Source: CAD feature listing. Evaluate the final solid. Frame: model axes, mm. Face numbers are marked on the shaded views. Give positions to 0.01 mm unless a question says otherwise; leave off trailing zeros. Loops run counter-clockwise (first coordinate to the right, second up) from the corner with the lowest first, then second, coordinate; pieces in that order, holes last. Notation, with made-up numbers: M 34.25,-1 L 80.25,-1 A12 cw 80.25,12 Z; hole C 36.5,36 d5. An arc over 180 degrees is marked long. Answer in a Markdown table with one row per item.
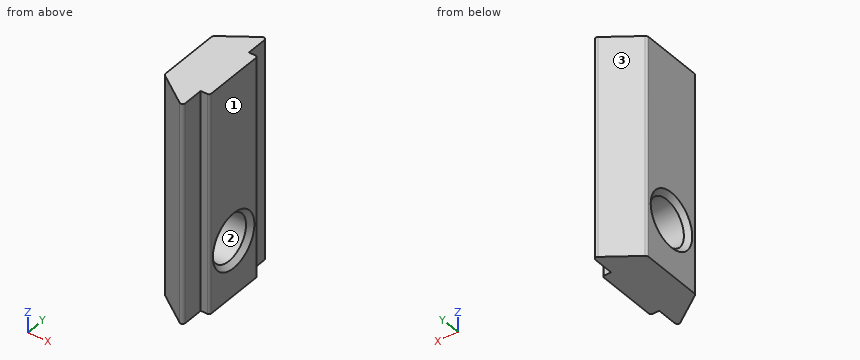
Autodesk Inventor part; units mm, degrees
ref_plane "nut_XY" through (0, 0, 0) normal (1, 0, 0) x (0, 0, -1)
ref_plane "nut_YZ" through (0, 0, 0) normal (0, 0, -1) x (0, 1, 0)
ref_plane "nut_ZX" through (0, 0, 0) normal (0, 1, 0) x (1, 0, 0)
sketch "Sketch_2" plane through (0, 0, 0) normal (0, 0, 1) x (1, 0, 0)
  arc A0 (-4.1, -2.7438) -> (-3.972, -2.9896) centre (-3.8, -2.7438) ccw
  line L0 (-3.972, -2.9896) -> (-1.1589, -4.9588)
  arc A1 (-1.1589, -4.9588) -> (-0.8, -4.7719) centre (-1.0281, -4.7719) ccw
  line L1 (-0.8, -4.7719) -> (-0.8, -2.9)
  line L2 (-0.8, -2.9) -> (-0.2, -2.9)
  arc A2 (-0.2, -2.9) -> (0, -2.7) centre (-0.2, -2.7) ccw
  line L3 (0, -2.7) -> (0, 2.7)
  arc A3 (0, 2.7) -> (-0.2, 2.9) centre (-0.2, 2.7) ccw
  line L4 (-0.2, 2.9) -> (-0.8, 2.9)
  line L5 (-0.8, 2.9) -> (-0.8, 4.7719)
  arc A4 (-0.8, 4.7719) -> (-1.1589, 4.9588) centre (-1.0281, 4.7719) ccw
  line L6 (-1.1589, 4.9588) -> (-3.972, 2.9896)
  arc A5 (-3.972, 2.9896) -> (-4.1, 2.7438) centre (-3.8, 2.7438) ccw
  line L7 (-4.1, 2.7438) -> (-4.1, -2.7438)
extrude "Extrusion1" add sketch "Sketch_2" along normal blind 15 and the other way blind 5
sketch "Sketch_5" plane through (0, 0, 0) normal (0, 0, 1) x (1, 0, 0)
  line L0 (0, 0) -> (-4.1, 0)
  line L1 (-4.1, 0) -> (-4.1, 2.5)
  line L2 (-4.1, 2.5) -> (-3.667, 2.067)
  line L3 (-3.667, 2.067) -> (-0.433, 2.067)
  line L4 (-0.433, 2.067) -> (0, 2.5)
  line L5 (0, 2.5) -> (0, 0)
  line L6 (0, 0) -> (-4.1, 0)
revolve "Revolution1" cut sketch "Sketch_5" angle 360 about axis through (0, 0, 0) along (1, 0, 0)
thread "Thread1"
ref_plane "nut_XY" through (0, 0, 0) normal (1, 0, 0) x (0, 0, -1)
ref_plane "nut_YZ" through (0, 0, 0) normal (0, 0, -1) x (0, 1, 0)
ref_plane "nut_ZX" through (0, 0, 0) normal (0, 1, 0) x (1, 0, 0)
ref_plane "to_bolt_XY" through (-4.1, 0, 0) normal (1, 0, 0) x (0, 0, -1)
ref_plane "to_bolt_YZ" through (-4.1, 0, 0) normal (0, 0, -1) x (0, 1, 0)
ref_plane "to_bolt_ZX" through (-4.1, 0, 0) normal (0, 1, 0) x (1, 0, 0)
ref_plane "to_frames_XY" through (-0.8, 0, 0) normal (1, 0, 0) x (0, 0, -1)
ref_plane "to_frames_YZ" through (-0.8, 0, 0) normal (0, 0, -1) x (0, 1, 0)
ref_plane "to_frames_ZX" through (-0.8, 0, 0) normal (0, 1, 0) x (1, 0, 0)
ref_plane "to_lane_XY" through (0, 0, 0) normal (0, 0, 1) x (1, 0, 0)
ref_plane "to_lane_YZ" through (0, 0, 0) normal (1, 0, 0) x (0, 1, 0)
ref_plane "to_lane_ZX" through (0, 0, 0) normal (0, 1, 0) x (0, 0, 1)
properties part number "HNTTSS5-5"
Q1. Section query B-B (z = 0). Output: boundary loops of the cut face in (x, y).
Values follow:
| item | result |
|---|---|
| outline | M -4.1,-2.74 A0.3 ccw -3.97,-2.99 L -1.16,-4.96 A0.23 ccw -0.8,-4.77 L -0.8,-2.9 L -0.2,-2.9 A0.2 ccw 0,-2.7 L 0,-2.5 L -0.43,-2.07 L -3.67,-2.07 L -4.1,-2.5 Z; M -4.1,2.5 L -3.67,2.07 L -0.43,2.07 L 0,2.5 L 0,2.7 A0.2 ccw -0.2,2.9 L -0.8,2.9 L -0.8,4.77 A0.23 ccw -1.16,4.96 L -3.97,2.99 A0.3 ccw -4.1,2.74 Z |
Q2. Section query D-D (x = -1.45). Output: boundary loops of the cut face in (y, z), plus the area to 3 significant figures.
Values follow:
| item | result |
|---|---|
| outline | M -4.76,-5 L 4.76,-5 L 4.76,15 L -4.76,15 Z; hole C 0,0 d4.13 |
| area | 177 mm^2 |
Q3. Contact query for flat-ended pins moving along their axis: pin 1 Ø2 at (x, y) = (-3.5, -4) entering from -Z; pin 2 Ø1.5 at (y, z) = (4, 5.5) entering from +X; pin 3 Ø1.5 at (x, z) = (-2, 11) entering from +Y (3 decimals); pin 4 Ø0.5 at (x, z) = (-0.5, 6) entering from +Y. Output: stop coordinate, or through.
Values follow:
| item | result |
|---|---|
| pin 1 | z = -5 |
| pin 2 | x = -0.8 |
| pin 3 | y = 4.895 |
| pin 4 | y = 2.9 |
Q4. Ray query, probe 1 along Z at (x, y) = (-2.45, 0); probe 2 along Y at (x, z) = (-0.65, 2.5); probe 3 along Z at (x, y) = (-1.05, 1). Return the intervals inside material, ascending. Write a range as from..to.
Values follow:
| item | result |
|---|---|
| probe 1 | -5..-2.07, 2.07..15 |
| probe 2 | -2.9..2.9 |
| probe 3 | -5..-1.81, 1.81..15 |
Q5. Mould query, pull axis Y, two halves, no side actions, for the marked faces 1, 2 and 3. Classes: +Y half, -Y half, draft (parallel to the pull), parting line (faces both ways), or undercut.
Values follow:
| item | result |
|---|---|
| face 1 | draft |
| face 2 | undercut |
| face 3 | +Y half |
Q6. Section query C-C (z = 9). Output: boundary loops of the cut face in (x, y), plus the area to 3 significant figures.
Values follow:
| item | result |
|---|---|
| outline | M -4.1,-2.74 A0.3 ccw -3.97,-2.99 L -1.16,-4.96 A0.23 ccw -0.8,-4.77 L -0.8,-2.9 L -0.2,-2.9 A0.2 ccw 0,-2.7 L 0,2.7 A0.2 ccw -0.2,2.9 L -0.8,2.9 L -0.8,4.77 A0.23 ccw -1.16,4.96 L -3.97,2.99 A0.3 ccw -4.1,2.74 Z |
| area | 31.3 mm^2 |
Q7. Section query A-A (y = 0). Output: boundary loops of the cut face in (x, z).
Values follow:
| item | result |
|---|---|
| outline | M -4.1,-5 L 0,-5 L 0,-2.5 L -0.43,-2.07 L -3.67,-2.07 L -4.1,-2.5 Z; M -4.1,2.5 L -3.67,2.07 L -0.43,2.07 L 0,2.5 L 0,15 L -4.1,15 Z |
